The model under review builds one solid part; all positions refer to its coordinate system, in mm. A direction names the side the tool comes from. Round coordinates to 2 decimals unless told otherwise and drop trailing zeros. Write each loop counter-clockwise with the first axis right and the second up, starting at its lowest first coordinate (ties: lowest second). Pieces come first, ordered by that corner, then holes. Notation, with made-up numbers: M 71,59.5 L 125,59.5 A23 cw 125,81.5 Z; hole C 22.25,74 d6. An arc over 180 degrees is marked long. One line per item, written item: value. Start each with the question number.
1) Mouldability with a two-part tool opening along X and no side actions: class faces 4 (the face through (3.233, -1.341, 0.294)), 5 (the face through (0.05, -0.21, -13.38)), 6 (the face through (0, -2, -21.5)) as +X half, -X half, draft (parallel to the pull), parting line (faces both ways), or undercut.
2) Tool access review of faces 1 (the face through (0, -2, 21.5)), 2 (the face through (-0.27, -1.22, -17.45)), 3 (the face through (0.27, -1.22, 17.45)): name each direction out of +Z, -Z, +X, -X, +Y, -Y from which nothing blocks a thin tool from reaching the whole face with its end or side.
3) Take a section at A-A, the plane z = -14.5. Write out the cut boundary in (x, y), and give its area (3 significant figures).
4) Wall thickness on probe 1 along Y at (x, z) = (0, 19.25); probe 2 along X at (y, z) = (-1.5, 14.5); probe 3 along Y at (x, z) = (-0.25, 6): over which ranges is each line inside the solid? List them lowest first.
5) For P1, Ø4, axis at x = 0, y = 0, coming from the -Z side; P2, Ø2, axis at x = -1.5, z = -0.5, coming from the +Y side; P3, Ø1, axis at x = 1.5, z = -13.5, coming from the -Y side; P4, Ø3, axis at y = 2.5, z = 4.5, coming from the -X side, all flat-tipped, find the tip position at first contact; note any pin that passes through.
6) Take a section at B-B, the plane z = -3. Write out the cut boundary in (x, y).
from build123d import *

# Parameters (mm, degrees)
SKETCH_1_R                       = 3.5
EXTRUDE_1_DEPTH                  = 21.5
HOLE_WIZARD_M3_1_D               = 2.5
HOLE_WIZARD_M3_1_DEPTH           = 7.5
HOLE_WIZARD_M3_1_TIP             = 0.751075774
HOLE_WIZARD_M3_1_ON_FACE_2_D     = 2.5
HOLE_WIZARD_M3_1_ON_FACE_2_DEPTH = 7.5
HOLE_WIZARD_M3_1_ON_FACE_2_TIP   = 0.751075774
CHAMFER_1_SIZE                   = 0.5


with BuildPart() as part:
    # 草图1 → 拉伸1 (new, symmetric)
    with BuildSketch(Plane.XY):
        Circle(SKETCH_1_R)
    extrude(amount=EXTRUDE_1_DEPTH, both=True)

    # M3 螺纹孔1
    with Locations(Plane.XY.offset(21.5)):
        with Locations((0, 0)):
            Hole(HOLE_WIZARD_M3_1_D / 2, depth=HOLE_WIZARD_M3_1_DEPTH)
            with Locations((0, 0, -(HOLE_WIZARD_M3_1_DEPTH + HOLE_WIZARD_M3_1_TIP / 2))):  # 118° drill point
                Cone(0, HOLE_WIZARD_M3_1_D / 2, HOLE_WIZARD_M3_1_TIP, mode=Mode.SUBTRACT)

    # M3 螺纹孔1 on face 2
    with Locations(Plane(origin=(0, 0, -21.5), x_dir=(-1, 0, 0), z_dir=(0, 0, -1))):
        with Locations((0, 0)):
            Hole(HOLE_WIZARD_M3_1_ON_FACE_2_D / 2, depth=HOLE_WIZARD_M3_1_ON_FACE_2_DEPTH)
            with Locations((0, 0, -(HOLE_WIZARD_M3_1_ON_FACE_2_DEPTH + HOLE_WIZARD_M3_1_ON_FACE_2_TIP / 2))):  # 118° drill point
                Cone(0, HOLE_WIZARD_M3_1_ON_FACE_2_D / 2, HOLE_WIZARD_M3_1_ON_FACE_2_TIP, mode=Mode.SUBTRACT)

    # 倒角1
    chamfer_1_edges = [part.edges().sort_by_distance(p)[0] for p in [
        (-3.5, 0, -21.5),
        (-3.5, 0, 21.5),
        (-1.25, 0, -21.5),
        (1.25, 0, 21.5),
    ]]
    chamfer(chamfer_1_edges, length=CHAMFER_1_SIZE)


solid = part.part
Checked values:
1. face 4: parting line
1. face 5: undercut
1. face 6: draft
2. face 1: +Z, +X, -X, +Y, -Y
2. face 2: -Z
2. face 3: +Z
3. outline: C 0,0 d7; hole C 0,0 d2.5
3. area: 33.6 mm2
4. probe 1: y = -3.5 to -1.25, 1.25 to 3.5
4. probe 2: x = -3.16 to 3.16
4. probe 3: y = -3.49 to 3.49
5. P1: stops at z = -21.5
5. P2: stops at y = 3.46
5. P3: stops at y = -3.35
5. P4: stops at x = -3.35
6. outline: C 0,0 d7
